from build123d import *

# Parameters (mm, degrees)
SKIZZE1_W                       = 20
SKIZZE1_H                       = 20
AUFSATZ_LINEAR_AUSTRAGEN1_DEPTH = 300
SKIZZE2_R                       = 3
SCHNITT_LINEAR_AUSTRAGEN1_DEPTH = 301.83217913
SKETCH1_R                       = 3
EXTRUDE1_DEPTH                  = 301.83217913


with BuildPart() as part:
    # Skizze1 → Aufsatz-Linear austragen1 (new body)
    with BuildSketch(Plane(origin=(0, 0, 0), x_dir=(0, 0, -1), z_dir=(1, 0, 0))):
        Rectangle(SKIZZE1_W, SKIZZE1_H)
    extrude(amount=AUFSATZ_LINEAR_AUSTRAGEN1_DEPTH)

    # Skizze2 → Schnitt-Linear austragen1 (cut, through all)
    with BuildSketch(Plane(origin=(0, 10, 0), x_dir=(1, 0, 0), z_dir=(0, 1, 0))):
        with Locations(Location((40, 0, 0), (0, 0, 270))):
            Circle(SKIZZE2_R)
        with Locations(Location((60, 0, 0), (0, 0, 270))):
            Circle(SKIZZE2_R)
        with Locations(Location((80, 0, 0), (0, 0, 270))):
            Circle(SKIZZE2_R)
    extrude(amount=-SCHNITT_LINEAR_AUSTRAGEN1_DEPTH, mode=Mode.SUBTRACT)

    # Sketch1 → Extrude1 (cut, through all)
    with BuildSketch(Plane.XY.offset(10)):
        with Locations((190, 0)):
            Circle(SKETCH1_R)
        with Locations((224.5, 0)):
            Circle(SKETCH1_R)
    extrude(amount=-EXTRUDE1_DEPTH, mode=Mode.SUBTRACT)


solid = part.part
Build history of the part. All positions in model axes, mm. Give positions to 0.01 mm unless a question says otherwise; leave off trailing zeros. Order: outer loops, then holes, each group sorted by start corner. A loop starts at its lowest first (then second) coordinate and runs counter-clockwise, first axis right, second up. Notation, with made-up numbers: M 19.5,53.25 L 34.5,53.25 A31 ccw 34.5,83.25 Z; hole C -8,82 d4. An arc over 180 degrees is marked long. Use one line per item in the form item = value.
1) Probe probe 1 along X at (y, z) = (4.75, 0); probe 2 along X at (y, z) = (2.75, -1); probe 3 along X at (y, z) = (-8, -2.25). List the from-to ranges inside material, lowest first.
Calculated:
probe_1 = 0 to 37, 43 to 57, 63 to 77, 83 to 300
probe_2 = 0 to 37.17, 42.83 to 57.17, 62.83 to 77.17, 82.83 to 188.8, 191.2 to 223.3, 225.7 to 300
probe_3 = 0 to 38.02, 41.98 to 58.02, 61.98 to 78.02, 81.98 to 300
2) Saw through at C-C (x = 40). Give the cut face in (y, z).
Calculated:
outline = M -10,-10 L 10,-10 L 10,-3 L -10,-3 Z; M -10,3 L 10,3 L 10,10 L -10,10 Z
3) Saw through at A-A (y = 0). Give the cut face in (x, z).
Calculated:
outline = M 0,-10 L 187,-10 L 187,10 L 0,10 Z; M 193,-10 L 221.5,-10 L 221.5,10 L 193,10 Z; M 227.5,-10 L 300,-10 L 300,10 L 227.5,10 Z; hole C 40,0 d6; hole C 60,0 d6; hole C 80,0 d6
4) Saw through at B-B (z = 0). Give the cut face in (x, y).
Calculated:
outline = M 0,-10 L 37,-10 L 37,10 L 0,10 Z; M 43,-10 L 57,-10 L 57,10 L 43,10 Z; M 63,-10 L 77,-10 L 77,10 L 63,10 Z; M 83,-10 L 300,-10 L 300,10 L 83,10 Z; hole C 190,0 d6; hole C 224.5,0 d6
5) Drop a flat-ended pin along its axis: pin 1 (9.5 mm diameter, centred on x = 60, z = 0, fed in from -Y). Give the stop position or say it passes through.
Calculated:
pin_1 = -10
6) Two-plate mould, pull along X, no slides. Class faces 1 (the face through (77.07, 0.14, -0.65)), 2 (the face through (300, 0, 0)), 3 (the face through (192.86, 0.9, 0.14)), 4 (the face through (148, 0, -10)): released by +X, released by -X, zero draft, split by the parting line, or undercut.
Calculated:
face_1 = undercut
face_2 = released by +X
face_3 = undercut
face_4 = zero draft
